Part model, mm, in its own coordinate system. A direction names the side the tool comes from. Give positions to 0.01 mm unless a question says otherwise; leave off trailing zeros. Order: outer loops, then holes, each group sorted by start corner. A loop starts at its lowest first (then second) coordinate and runs counter-clockwise, first axis right, second up.
1. Drop flat-ended pins along their axis: pin 1 Ø5 at (y, z) = (22, -30) entering from +X; pin 2 Ø4 at (y, z) = (27.5, -27.5) entering from -X. Give the stop position or say it passes through.
2. Which spindle directions (+Z, -Z, +X, -X, +Y, -Y) get a long thin tool onto all of the face, cutting with end or side? Do faces 4 (the cylindrical face through (3, 6, -25.5)), 5 (the flat face through (19, 18, 0)). Say none if no direction does.
3. Mould opens along Y. For faces 1 (the flat face through (21, 0, 1)), 2 (the cylindrical face through (3.04, 29.61, -8.84)), 3 (the flat face through (19, 18, 10)) say: +Y half, -Y half, draft (parallel to the pull), parting line (faces both ways), or undercut.
4. Slice it at A-A on x = 32.5. List the corners of the cut face in (y, z), and give its area (3 significant figures).
5. Slice it at C-C on x = 4.5. List the corners of the cut face in (y, z).
6. Slice it at B-B on z = -7.5. List the corners of the cut face in (x, y).
7. Probe line 1 (Y direction, x = 2.85, z = -27.5); line 2 (X direction, y = 17, z = 2); line 3 (Y direction, x = 3, z = -7). List the from-to ranges inside material, lowest first.
8. Slice it at D-D on y = 7.5. List the corners of the cut face in (x, z), and give its area (3 significant figures).
from build123d import *

# Parameters (mm, degrees)
SKETCH1_W           = 50
SKETCH1_H           = 35
SKETCH1_R           = 11
BOSS_EXTRUDE3_DEPTH = 10
BOSS_EXTRUDE6_DEPTH = 35
SKETCH9_R           = 2.5
CUT_EXTRUDE1_DEPTH  = 10
FILLET1_R           = 2


with BuildPart() as part:
    # Sketch1 → Boss-Extrude3 (new body)
    with BuildSketch(Plane.XY):
        with Locations((25, 17.5)):
            Rectangle(SKETCH1_W, SKETCH1_H)
        with Locations((32.5, 17.5)):
            Circle(SKETCH1_R, mode=Mode.SUBTRACT)
    extrude(amount=BOSS_EXTRUDE3_DEPTH)

    # Sketch8 → Boss-Extrude6 (add)
    with BuildSketch(Plane(origin=(0, 0, 0), x_dir=(-1, 0, 0), z_dir=(0, 0, -1))):
        Polygon((-6, 10.000000197), (-6, 0), (0, 0), (0, 10.000000197), (0, 25), (0, 35), (-6, 35), (-6, 25), align=None)
    extrude(amount=BOSS_EXTRUDE6_DEPTH)

    # Sketch9 → Cut-Extrude1 (cut)
    with BuildSketch(Plane(origin=(6, 0, 0), x_dir=(0, 0, -1), z_dir=(1, 0, 0))):
        with Locations((7.5, 27.5)):
            Circle(SKETCH9_R)
        with Locations((27.5, 27.5)):
            Circle(SKETCH9_R)
        with Locations((7.5, 7.5)):
            Circle(SKETCH9_R)
        with Locations((27.5, 7.5)):
            Circle(SKETCH9_R)
    extrude(amount=-CUT_EXTRUDE1_DEPTH, mode=Mode.SUBTRACT)

    # Fillet1
    fillet1_edges = [part.edges().sort_by_distance(p)[0] for p in [
        (6, 17.5, 0),
    ]]
    fillet(fillet1_edges, radius=FILLET1_R)


solid = part.part
Data:
1. pin 1: stops at x = 6
1. pin 2: passes through
2. face 4: +X, -X
2. face 5: -Z, +X, +Y, -Y
3. face 1: -Y half
3. face 2: undercut
3. face 3: draft
4. outline: (0, 0) - (6.5, 0) - (6.5, 10) - (0, 10) - close; (28.5, 0) - (35, 0) - (35, 10) - (28.5, 10) - close
4. area: 130 mm2
5. outline: (0, -35) - (35, -35) - (35, 10) - (0, 10) - close; hole circle Ø5 at (7.5, -27.5); hole circle Ø5 at (7.5, -7.5); hole circle Ø5 at (27.5, -27.5); hole circle Ø5 at (27.5, -7.5)
6. outline: (0, 0) - (6, 0) - (6, 5) - (0, 5) - close; (0, 10) - (6, 10) - (6, 25) - (0, 25) - close; (0, 30) - (6, 30) - (6, 35) - (0, 35) - close
7. line 1: y = 0 to 5, 10 to 25, 30 to 35
7. line 2: x = 0 to 21.51, 43.49 to 50
7. line 3: y = 0 to 5.05, 9.95 to 25.05, 29.95 to 35
8. outline: (0, -35) - (6, -35) - (6, -30) - (0, -30) - close; (0, -25) - (6, -25) - (6, -10) - (0, -10) - close; (0, -5) - (6, -5) - (6, -2) arc R2 cw to (8, 0) - (27.92, 0) - (27.92, 10) - (0, 10) - close; (37.08, 0) - (50, 0) - (50, 10) - (37.08, 10) - close
8. area: 559 mm2
